Source: CAD feature listing. Evaluate the final solid. Frame: model axes, mm. A direction names the side the tool comes from. Coordinates: 2 decimals unless noted, no trailing zeros. Loops run counter-clockwise (first coordinate to the right, second up) from the corner with the lowest first, then second, coordinate; pieces in that order, holes last. Notation, with made-up numbers: (18.5, -36.5) -> (71.5, -36.5) arc R20 cw to (71.5, -27.5) -> close; hole circle Ø11 at (23, 68). An arc over 180 degrees is marked (long way). Answer as a JSON object with one key per item and string values. Group by question number.
from build123d import *

# Parameters (mm, degrees)
F1_DEPTH = 6
F0_W     = 180
F0_H     = 70
F2_DEPTH = 3
F3_DEPTH = 6
F4_DEPTH = 6
F5_R     = 5


with BuildPart() as f1:
    # F0 (on Front) → F1 (new body)
    with BuildSketch(Plane.XZ):
        Polygon((-19.6854011617, -19.1057036918), (-7.0193172456, -19.1057036918), (-7.0193172456, 40.8025130914), (-19.6854011617, 40.8025130914), (-19.6854011617, 17.319121483), (-43.4048067561, 17.319121483), (-43.4048067561, 40.8025130914), (-56.1102263365, 40.8025130914), (-56.1102263365, -19.1057036918), (-43.4048067561, -19.1057036918), (-43.4048067561, 6.7509396648), (-19.6854011617, 6.7509396648), align=None)
    extrude(amount=F1_DEPTH)

    # F0 (on Front) → F2 (join)
    with BuildSketch(Plane.XZ):
        with Locations((26.3504379991, 11.104086518)):
            Rectangle(F0_W, F0_H)
        Polygon((-7.0193172456, 40.8025130914), (-7.0193172456, -19.1057036918), (-19.6854011617, -19.1057036918), (-19.6854011617, 6.7509396648), (-43.4048067561, 6.7509396648), (-43.4048067561, -19.1057036918), (-56.1102263365, -19.1057036918), (-56.1102263365, 40.8025130914), (-43.4048067561, 40.8025130914), (-43.4048067561, 17.319121483), (-19.6854011617, 17.319121483), (-19.6854011617, 40.8025130914), align=None, mode=Mode.SUBTRACT)
        with BuildLine():
            Line((44.1957177194, 40.8025130914), (56.8618016355, 40.8025130914))
            Line((56.8618016355, 40.8025130914), (56.8618016355, 2.0437718327))
            add(Edge.make_bspline(
                [(56.8618016355, 2.0437718327), (56.8618016355, -4.6039554401), (53.8919589781, -9.5995848107)],
                knots=[0, 0, 0, 1, 1, 1], degree=2))
            add(Edge.make_bspline(
                [(53.8919589781, -9.5995848107), (50.9221163208, -14.5952141813), (45.3036722649, -17.2634834121)],
                knots=[0, 0, 0, 1, 1, 1], degree=2))
            add(Edge.make_bspline(
                [(45.3036722649, -17.2634834121), (39.6852282089, -19.9317526429), (32.0278855516, -19.9317526429)],
                knots=[0, 0, 0, 1, 1, 1], degree=2))
            add(Edge.make_bspline(
                [(32.0278855516, -19.9317526429), (20.476312125, -19.9317526429), (14.0842666704, -14.0051792163)],
                knots=[0, 0, 0, 1, 1, 1], degree=2))
            add(Edge.make_bspline(
                [(14.0842666704, -14.0051792163), (7.6922212159, -8.0786057897), (7.6922212159, 2.20111449)],
                knots=[0, 0, 0, 1, 1, 1], degree=2))
            Line((7.6922212159, 2.20111449), (7.6922212159, 40.8025130914))
            Line((7.6922212159, 40.8025130914), (20.3451932439, 40.8025130914))
            Line((20.3451932439, 40.8025130914), (20.3451932439, 4.1285620424))
            add(Edge.make_bspline(
                [(20.3451932439, 4.1285620424), (20.3451932439, -2.7945148806), (23.1314694677, -6.0331512443)],
                knots=[0, 0, 0, 1, 1, 1], degree=2))
            add(Edge.make_bspline(
                [(23.1314694677, -6.0331512443), (25.9177456914, -9.2717876079), (32.3556827544, -9.2717876079)],
                knots=[0, 0, 0, 1, 1, 1], degree=2))
            add(Edge.make_bspline(
                [(32.3556827544, -9.2717876079), (38.5838296075, -9.2717876079), (41.3897736635, -6.0134834121)],
                knots=[0, 0, 0, 1, 1, 1], degree=2))
            add(Edge.make_bspline(
                [(41.3897736635, -6.0134834121), (44.1957177194, -2.7551792163), (44.1957177194, 4.2072333711)],
                knots=[0, 0, 0, 1, 1, 1], degree=2))
            Line((44.1957177194, 4.2072333711), (44.1957177194, 40.8025130914))
        make_face(mode=Mode.SUBTRACT)
        Polygon((94.6502631739, 30.2343312732), (94.6502631739, -19.1057036918), (81.9448435935, -19.1057036918), (81.9448435935, 30.2343312732), (65.6729904467, 30.2343312732), (65.6729904467, 40.8025130914), (110.9090044327, 40.8025130914), (110.9090044327, 30.2343312732), align=None, mode=Mode.SUBTRACT)
    extrude(amount=F2_DEPTH)

    # F0 (on Front) → F3 (join)
    with BuildSketch(Plane.XZ):
        with BuildLine():
            Line((56.8618016355, 2.0437718327), (56.8618016355, 40.8025130914))
            Line((56.8618016355, 40.8025130914), (44.1957177194, 40.8025130914))
            Line((44.1957177194, 40.8025130914), (44.1957177194, 4.2072333711))
            add(Edge.make_bspline(
                [(41.3897736635, -6.0134834121), (44.1957177194, -2.7551792163), (44.1957177194, 4.2072333711)],
                knots=[0, 0, 0, 1, 1, 1], degree=2))
            add(Edge.make_bspline(
                [(32.3556827544, -9.2717876079), (38.5838296075, -9.2717876079), (41.3897736635, -6.0134834121)],
                knots=[0, 0, 0, 1, 1, 1], degree=2))
            add(Edge.make_bspline(
                [(23.1314694677, -6.0331512443), (25.9177456914, -9.2717876079), (32.3556827544, -9.2717876079)],
                knots=[0, 0, 0, 1, 1, 1], degree=2))
            add(Edge.make_bspline(
                [(20.3451932439, 4.1285620424), (20.3451932439, -2.7945148806), (23.1314694677, -6.0331512443)],
                knots=[0, 0, 0, 1, 1, 1], degree=2))
            Line((20.3451932439, 4.1285620424), (20.3451932439, 40.8025130914))
            Line((20.3451932439, 40.8025130914), (7.6922212159, 40.8025130914))
            Line((7.6922212159, 40.8025130914), (7.6922212159, 2.20111449))
            add(Edge.make_bspline(
                [(14.0842666704, -14.0051792163), (7.6922212159, -8.0786057897), (7.6922212159, 2.20111449)],
                knots=[0, 0, 0, 1, 1, 1], degree=2))
            add(Edge.make_bspline(
                [(32.0278855516, -19.9317526429), (20.476312125, -19.9317526429), (14.0842666704, -14.0051792163)],
                knots=[0, 0, 0, 1, 1, 1], degree=2))
            add(Edge.make_bspline(
                [(45.3036722649, -17.2634834121), (39.6852282089, -19.9317526429), (32.0278855516, -19.9317526429)],
                knots=[0, 0, 0, 1, 1, 1], degree=2))
            add(Edge.make_bspline(
                [(53.8919589781, -9.5995848107), (50.9221163208, -14.5952141813), (45.3036722649, -17.2634834121)],
                knots=[0, 0, 0, 1, 1, 1], degree=2))
            add(Edge.make_bspline(
                [(56.8618016355, 2.0437718327), (56.8618016355, -4.6039554401), (53.8919589781, -9.5995848107)],
                knots=[0, 0, 0, 1, 1, 1], degree=2))
        make_face()
    extrude(amount=F3_DEPTH)

    # F0 (on Front) → F4 (join)
    with BuildSketch(Plane.XZ):
        Polygon((81.9448435935, -19.1057036918), (94.6502631739, -19.1057036918), (94.6502631739, 30.2343312732), (110.9090044327, 30.2343312732), (110.9090044327, 40.8025130914), (65.6729904467, 40.8025130914), (65.6729904467, 30.2343312732), (81.9448435935, 30.2343312732), align=None)
    extrude(amount=F4_DEPTH)

    # F5
    f5_edges = [f1.edges().sort_by_distance(p)[0] for p in [
        (-63.649562, -1.5, 46.104087),
        (116.350438, -1.5, 46.104087),
        (-63.649562, -1.5, -23.895913),
        (116.350438, -1.5, -23.895913),
    ]]
    fillet(f5_edges, radius=F5_R)


solid = f1.part
1. Section query D-D on x = 2. Return loops of the section in (y, z).
2. Ray query, L1, parallel to X at y = -3.25, z = 17; L2, parallel to X at y = -5, z = 23; L3, parallel to X at y = -5.5, z = 0.5. Return the intervals inside material, ascending.
3. Reachability of faces 1 (the face through (14, -4, 40.803)), 2 (the face through (74, -4, 30.234)), 3 (the face through (-7.019, -4, 10)) from +Z, -Z, +X, -X, +Y, -Y: full face, straight path, thin tool, end or side. Return the list, or none.
4. Mould query, pull axis X, two halves, no side actions, for faces 4 (the face through (114.847, -1.521, 44.678)), 5 (the face through (-43.405, -4, -6)), 6 (the face through (88, -4, -19.106)), 7 (the face through (-62.224, -1.521, -22.392)). Classes: pulls with the +X half, pulls with the -X half, needs draft (parallel to the pull), parting line crosses it, or undercut.
5. Pin query (flat end, axial travel): pin 1 Ø3.5 at (y, z) = (-5, 1) entering from +X; pin 2 Ø1.5 at (x, y) = (48.5, -4) entering from +Z; pin 3 Ø1.5 at (x, z) = (-2.5, -15.5) entering from -Y. Return the tip coordinate at first contact, or that it passes through.
6. Section query B-B on x = -30. Return loops of the section in (y, z), then the cut area to 3 significant figures.
7. Section query A-A on z = 33.5. Return loops of the section in (x, y).
8. Section query C-C on y = -4. State how many separate pieces and enclosed holes the cut face has, then the cut area to 3 significant figures.
Solved:
{
 "1": {"outline": "(-3, -23.9) -> (0, -23.9) -> (0, 46.1) -> (-3, 46.1) -> close"},
 "2": {"L1": "-56.11 to -7.02, 7.69 to 20.35, 44.2 to 56.86, 81.94 to 94.65", "L2": "-56.11 to -43.4, -19.69 to -7.02, 7.69 to 20.35, 44.2 to 56.86, 81.94 to 94.65", "L3": "-56.11 to -43.4, -19.69 to -7.02, 7.74 to 20.57, 43.96 to 56.82, 81.94 to 94.65"},
 "3": {"face 1": "+Z, +X, -X, -Y", "face 2": "-Z, -Y", "face 3": "+Z, -Z, -Y"},
 "4": {"face 4": "pulls with the +X half", "face 5": "undercut", "face 6": "needs draft", "face 7": "pulls with the -X half"},
 "5": {"pin 1": "x = 94.65", "pin 2": "z = 40.8", "pin 3": "y = -3"},
 "6": {"outline": "(-6, 6.75) -> (-3, 6.75) -> (-3, -23.9) -> (0, -23.9) -> (0, 46.1) -> (-3, 46.1) -> (-3, 17.32) -> (-6, 17.32) -> close", "area": "242 mm^2"},
 "7": {"outline": "(-63.65, -3) -> (-56.11, -3) -> (-56.11, -6) -> (-43.4, -6) -> (-43.4, -3) -> (-19.69, -3) -> (-19.69, -6) -> (-7.02, -6) -> (-7.02, -3) -> (7.69, -3) -> (7.69, -6) -> (20.35, -6) -> (20.35, -3) -> (44.2, -3) -> (44.2, -6) -> (56.86, -6) -> (56.86, -3) -> (65.67, -3) -> (65.67, -6) -> (110.91, -6) -> (110.91, -3) -> (116.35, -3) -> (116.35, 0) -> (-63.65, 0) -> close"},
 "8": {"separate pieces": "3", "enclosed holes": "0", "area": "4,520 mm^2"}
}
